```python
from build123d import *

# Parameters (mm, degrees)
F1_DEPTH = 1.3
F3_DEPTH = 4
F4_SIZE  = 0.5
F5_SIZE  = 3
F6_R     = 1.5
F8_D     = 2.7


with BuildPart() as f1:
    # F0 (on Top) → F1 (new body)
    with BuildSketch(Plane.XY):
        Polygon((-7.25, -7), (-0.25, -7), (7, 0.25), (7, 7.25), (-0.5, 7.25), (-0.5, 0.5), (-7.25, 0.5), align=None)
    extrude(amount=F1_DEPTH)

    # F2 (on face) → F3 (join)
    with BuildSketch(Plane(origin=(0, 0, 0), x_dir=(1, 0, 0), z_dir=(0, 0, -1))):
        Polygon((7, -5.75), (7, -0.25), (-0.25, 7), (-5.75, 7), (-5.75, 10), (-11.25, 10), (-11.25, 2), (-7.25, 2), (-7.25, -0.5), (-0.5, -0.5), (-0.5, -7.25), (2, -7.25), (2, -11.25), (10, -11.25), (10, -5.75), align=None)
    extrude(amount=F3_DEPTH)

    # F4
    f4_edges = [f1.edges().sort_by_distance(p)[0] for p in [
        (-5.75, -10, -2),
        (-11.25, -10, -2),
        (-7.25, -7, 0.65),
        (-11.25, -2, -2),
        (-7.25, 0.5, -1.35),
        (-0.5, 7.25, -1.35),
        (2, 11.25, -2),
        (7, 7.25, 0.65),
        (10, 11.25, -2),
        (10, 5.75, -2),
    ]]
    chamfer(f4_edges, length=F4_SIZE)

    # F5
    f5_edges = [f1.edges().sort_by_distance(p)[0] for p in [
        (-0.5, 0.5, -1.35),
    ]]
    chamfer(f5_edges, length=F5_SIZE)

    # F6
    f6_edges = [f1.edges().sort_by_distance(p)[0] for p in [
        (2, 9, 0),
        (-9, -2, 0),
    ]]
    fillet(f6_edges, radius=F6_R)

    # F8 (through all)
    with Locations(Plane.XY.offset(1.3)):
        with Locations((3.5, 3.25), (-3.25, -3.5)):
            Hole(F8_D / 2)


solid = f1.part
```
Work out the finished part from the listing and answer in its coordinate system (mm). A direction names the side the tool comes from. Give positions to 0.01 mm unless a question says otherwise; leave off trailing zeros. Loops run counter-clockwise (first coordinate to the right, second up) from the corner with the lowest first, then second, coordinate; pieces in that order, holes last. Notation, with made-up numbers: (-29.75, 43.25) - (-20.75, 43.25) arc R17 cw to (-20.75, 61.25) - close; hole circle Ø8 at (54, 79). An arc over 180 degrees is marked (long way). One line per question, with ' | ' between items.
(1) A tool of negligible diameter and unlimited length cuts with its end or side. For faces 1 (the face through (-7.25, -1.9, -0.7)), 2 (the face through (8, 5.75, -2)), 3 (the face through (2, 9, -3)), 4 (the face through (7, 9, 0)), from which of +Z, -Z, +X, -X, +Y, -Y can it reach the whole face along a straight path? Write none if from no direction.
Recorded:
face 1: +Z, -X, +Y | face 2: +Z, -Z, +X, -Y | face 3: +Z, -Z, -X, +Y | face 4: +Z, +X, +Y
(2) The part is cut by section D-D (y = 6). Write down the section's boundary in (x, z).
Recorded:
outline: (-0.5, -4) - (9.75, -4) - (9.75, 0) - (7, 0) - (7, 1.3) - (-0.5, 1.3) - close
(3) Each of these flat-tipped pins is pushed along its axis until it touches: pin 1 Ø3 at (x, y) = (7.5, 7.5) entering from +Z; pin 2 Ø2.5 at (y, z) = (5, -1) entering from -X; pin 3 Ø2 at (y, z) = (8.5, -3) entering from -X; pin 4 Ø2 at (y, z) = (-7.5, -2) entering from +X. Where does it stop, or does it pass through?
Recorded:
pin 1: stops at z = 1.3 | pin 2: stops at x = -0.5 | pin 3: stops at x = 2 | pin 4: stops at x = 0.25
(4) Straight lines are drawn through the part: probe 1 along Y at (x, z) = (3.5, -2); probe 2 along Y at (x, z) = (6.5, -0.35); probe 3 along Z at (x, y) = (-9, -7.5). For each, find the intervals that lie inside material, in ascending order.
Recorded:
probe 1: y = -3.25 to 1.9, 4.6 to 11.25 | probe 2: y = -0.25 to 11.25 | probe 3: z = -4 to 0
(5) The part is cut by section C-C (y = 3.25). Write down the section's boundary in (x, z).
Recorded:
outline: (-0.75, -4) - (2.15, -4) - (2.15, 1.3) - (-0.75, 1.3) - close; (4.85, -4) - (7, -4) - (7, 1.3) - (4.85, 1.3) - close
(6) The part is cut by section B-B (z = 0.75). Write down the section's boundary in (x, y).
Recorded:
outline: (-7.25, -6.5) - (-6.75, -7) - (-0.25, -7) - (7, 0.25) - (7, 6.75) - (6.5, 7.25) - (0, 7.25) - (-0.5, 6.75) - (-0.5, 3.5) - (-3.5, 0.5) - (-6.75, 0.5) - (-7.25, 0) - close; hole circle Ø2.7 at (-3.25, -3.5); hole circle Ø2.7 at (3.5, 3.25)
(7) The part is cut by section A-A (x = -3.25). Write down the section's boundary in (y, z), then the cut area to 3 significant figures.
Recorded:
outline: (-7, -4) - (-4.85, -4) - (-4.85, 1.3) - (-7, 1.3) - close; (-2.15, -4) - (0.75, -4) - (0.75, 1.3) - (-2.15, 1.3) - close | area: 26.8 mm²
(8) The mould has two halves that part along X. Classify faces 5 (the face through (-4.497, -4.017, -1.387)), 6 (the face through (-2, 2, -1)), 7 (the face through (-5.75, -8, -2)), 8 (the face through (0, 0, 1.3)): +X half, -X half, draft (parallel to the pull), parting line (faces both ways), or undercut.
Recorded:
face 5: undercut | face 6: -X half | face 7: +X half | face 8: draft
